```python
from build123d import *

# Parameters (mm, degrees)
SKETCH_1_R          = 12
EXTRUDE_1_DEPTH     = 30
CUT_EXTRUDE_START   = -7.5
SKETCH_2_R          = 12
CUT_EXTRUDE_1_DEPTH = 7.5
CUT_EXTRUDE_2_DEPTH = 7.5
SKETCH_4_W          = 642
SKETCH_4_H          = 50
CUT_EXTRUDE_3_DEPTH = 12.5
SKETCH_5_W          = 642
SKETCH_5_H          = 50
CUT_EXTRUDE_4_DEPTH = 12.5


with BuildPart() as part:
    # 草图1 → 凸台-拉伸1 (new body)
    with BuildSketch(Plane.XY):
        with BuildLine():
            Line((675.999999195, -9.999997784), (706.830258378, 1.202458393))
            ThreePointArc((706.830258378, 1.202458393), (720, 20), (706.830258378, 38.797541607))
            Line((706.830258378, 38.797541607), (675.999999195, 49.999997784))
            Line((675.999999195, 49.999997784), (24.000000805, 49.999997784))
            Line((24.000000805, 49.999997784), (-6.830258378, 38.797541607))
            ThreePointArc((-6.830258378, 38.797541607), (-20, 20), (-6.830258378, 1.202458393))
            Line((-6.830258378, 1.202458393), (24.000000805, -9.999997784))
            Line((24.000000805, -9.999997784), (675.999999195, -9.999997784))
        make_face()
        with Locations((0, 20)):
            Circle(SKETCH_1_R, mode=Mode.SUBTRACT)
        with Locations(Location((700, 20, 0), (0, 0, 180))):
            Circle(SKETCH_1_R, mode=Mode.SUBTRACT)
    extrude(amount=EXTRUDE_1_DEPTH)

    # 草图2 → 切除-拉伸1 (cut)
    # profile 1 of 2: a face of its own
    with BuildSketch(Plane.XY.offset(30).offset(CUT_EXTRUDE_START)):
        with BuildLine():
            Line((24.000000805, 49.999997784), (-6.830258378, 38.797541607))
            ThreePointArc((-6.830258378, 38.797541607), (-20, 20), (-6.830258378, 1.202458393))
            Line((-6.830258378, 1.202458393), (24.000000805, -9.999997784))
            Line((24.000000805, -9.999997784), (24.000000805, 49.999997784))
        make_face()
        with Locations((0, 20)):
            Circle(SKETCH_2_R, mode=Mode.SUBTRACT)
    # profile 2 of 2: a face of its own
    with BuildSketch(Plane.XY.offset(30).offset(CUT_EXTRUDE_START)):
        with BuildLine():
            Line((706.830258378, 38.797541607), (675.999999195, 49.999997784))
            Line((675.999999195, 49.999997784), (675.999999195, -9.999997784))
            Line((675.999999195, -9.999997784), (706.830258378, 1.202458393))
            ThreePointArc((706.830258378, 1.202458393), (720, 20), (706.830258378, 38.797541607))
        make_face()
    extrude(amount=CUT_EXTRUDE_1_DEPTH, mode=Mode.SUBTRACT)

    # 草图3 → 切除-拉伸2 (cut)
    with BuildSketch(Plane(origin=(0, 0, 0), x_dir=(-1, 0, 0), z_dir=(0, 0, -1))):
        with BuildLine():
            Line((6.830258378, 38.797541607), (-24.000000805, 49.999997784))
            Line((-24.000000805, 49.999997784), (-24.000000805, -9.999997784))
            Line((-24.000000805, -9.999997784), (6.830258378, 1.202458393))
            ThreePointArc((6.830258378, 1.202458393), (20, 20), (6.830258378, 38.797541607))
        make_face()
        with BuildLine():
            Line((-706.830258378, 38.797541607), (-675.999999195, 49.999997784))
            Line((-675.999999195, 49.999997784), (-675.999999195, -9.999997784))
            Line((-675.999999195, -9.999997784), (-706.830258378, 1.202458393))
            ThreePointArc((-706.830258378, 1.202458393), (-720, 20), (-706.830258378, 38.797541607))
        make_face()
    extrude(amount=-CUT_EXTRUDE_2_DEPTH, mode=Mode.SUBTRACT)

    # 草图4 → 切除-拉伸3 (cut)
    with BuildSketch(Plane(origin=(0, 0, 0), x_dir=(-1, 0, 0), z_dir=(0, 0, -1))):
        with Locations((-349.999999195, 20.000002216)):
            Rectangle(SKETCH_4_W, SKETCH_4_H)
    extrude(amount=-CUT_EXTRUDE_3_DEPTH, mode=Mode.SUBTRACT)

    # 草图5 → 切除-拉伸4 (cut)
    with BuildSketch(Plane.XY.offset(30)):
        with Locations((350.000000805, 19.999997784)):
            Rectangle(SKETCH_5_W, SKETCH_5_H)
    extrude(amount=-CUT_EXTRUDE_4_DEPTH, mode=Mode.SUBTRACT)


solid = part.part
```
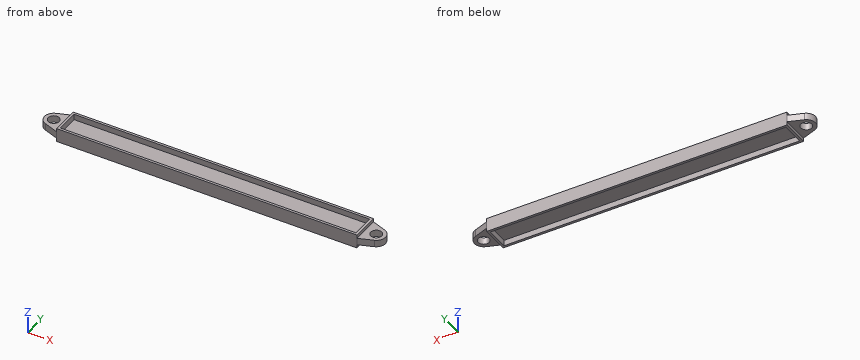
Design review of the part built by this model. Coordinates are the model's own, in mm. Round coordinates to 2 decimals unless told otherwise and drop trailing zeros. Write each loop counter-clockwise with the first axis right and the second up, starting at its lowest first coordinate (ties: lowest second). Pieces come first, ordered by that corner, then holes. Notation, with made-up numbers: (-26.5, 61.25) -> (-22.5, 61.25) arc R26 ccw to (-22.5, 79.25) -> close; hole circle Ø5 at (20.25, 41.25). An arc over 180 degrees is marked (long way). Answer in a Markdown table with one row per item.
Q1. Take a section at C-C, the plane x = 700. State the section outline as (y, z) points, then the cut area to 3 significant figures.
The answers:
| item | result |
|---|---|
| outline | (-1.28, 7.5) -> (8, 7.5) -> (8, 22.5) -> (-1.28, 22.5) -> close; (32, 7.5) -> (41.28, 7.5) -> (41.28, 22.5) -> (32, 22.5) -> close |
| area | 278 mm² |
Q2. Clearance check with flat-ended pins moving along their axes: pin 1 Ø14 at (y, z) = (20, 3.5) entering from +X; pin 2 Ø10 at (y, z) = (32.5, 6) entering from +X; pin 3 Ø10 at (y, z) = (12.5, 26) entering from -X; pin 4 Ø8 at (y, z) = (26.5, 2.5) entering from -X. State where each tip first meets the part, or that it passes through.
The answers:
| item | result |
|---|---|
| pin 1 | x = 720 |
| pin 2 | x = 718.45 |
| pin 3 | x = -19.61 |
| pin 4 | x = 24 |
Q3. Take a section at B-B, the plane x = 517.5. State the section outline as (y, z) points.
The answers:
| item | result |
|---|---|
| outline | (-10, 0) -> (-5, 0) -> (-5, 12.5) -> (45, 12.5) -> (45, 0) -> (50, 0) -> (50, 30) -> (45, 30) -> (45, 17.5) -> (-5, 17.5) -> (-5, 30) -> (-10, 30) -> close |
Q4. To check wall thickness, follow L1, parallel to Y at x = 670, z = 26.75; L2, parallel to X at y = 19, z = 2; L3, parallel to X at y = 27, z = 19.5 (3 decimals). State the ranges of each line that lie inside material, in increasing order. Write a range as [from, to].
The answers:
| item | result |
|---|---|
| L1 | [-10, -5], [45, 50] |
| L2 | [24, 29], [671, 676] |
| L3 | [-18.735, -9.747], [9.747, 29], [671, 690.253], [709.747, 718.735] |
Q5. Take a section at A-A, the plane y = 20. State the section outline as (x, z) points, then the cut area to 3 significant figures.
The answers:
| item | result |
|---|---|
| outline | (-20, 7.5) -> (-12, 7.5) -> (-12, 22.5) -> (-20, 22.5) -> close; (12, 7.5) -> (24, 7.5) -> (24, 0) -> (29, 0) -> (29, 12.5) -> (671, 12.5) -> (671, 0) -> (676, 0) -> (676, 7.5) -> (688, 7.5) -> (688, 22.5) -> (676, 22.5) -> (676, 30) -> (671, 30) -> (671, 17.5) -> (29, 17.5) -> (29, 30) -> (24, 30) -> (24, 22.5) -> (12, 22.5) -> close; (712, 7.5) -> (720, 7.5) -> (720, 22.5) -> (712, 22.5) -> close |
| area | 4,110 mm² |
